Can you work these out from the drawing? Everything is in mm from the part's minimum corner. Coordinates: 2 decimals unless noted, no trailing zeros. Loops run counter-clockwise (first coordinate to the right, second up) from the corner with the lowest first, then second, coordinate; pieces in that order, holes last.
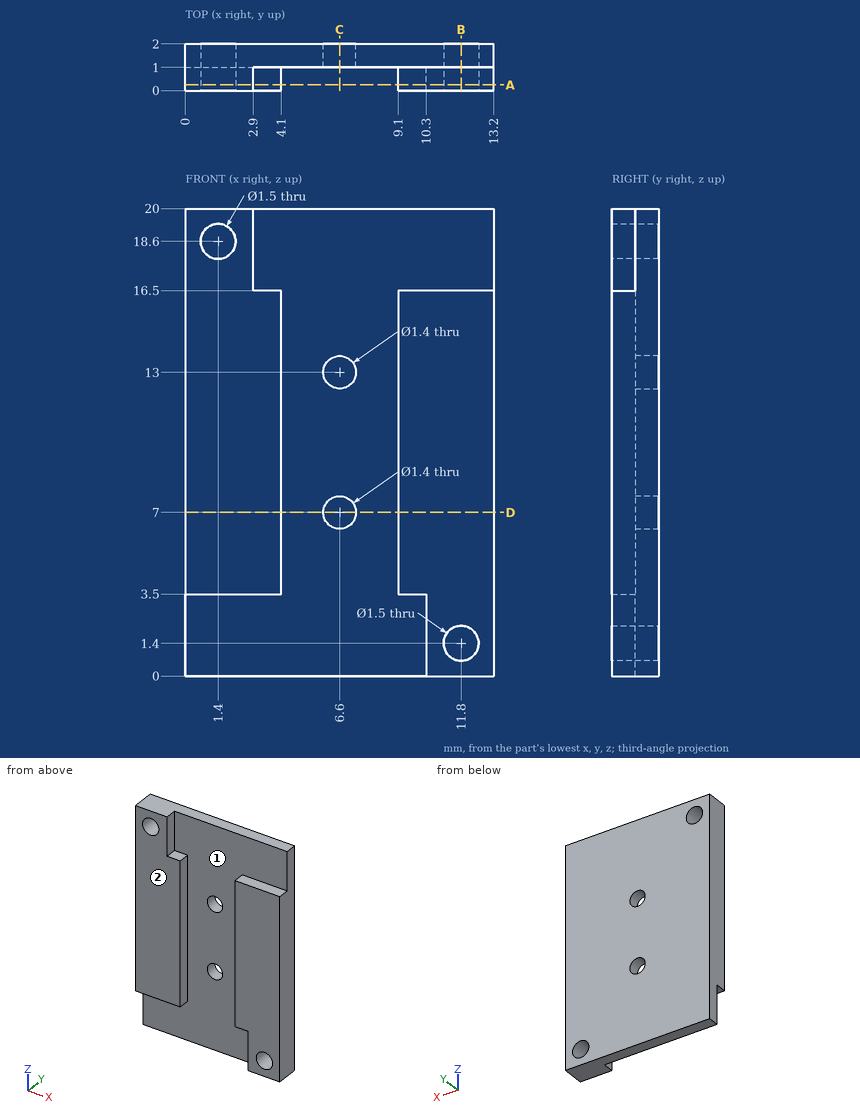
(1) For pin 1 (0.5 mm diameter, centred on y = 0.5, z = 2, fed in from -X); pin 2 (1.3 mm diameter, centred on x = 6.6, z = 7, fed in from +Y); pin 3 (0.5 mm diameter, centred on y = 0.5, z = 18.5, fed in from +X); pin 4 (0.5 mm diameter, centred on x = 11, y = 0.5, fed in from +Z), each with a flat end and sliding along its axis, tell me the tip position at first contact or that it passes through.
Answers:
pin 1: stops at x = 10.3
pin 2: passes through
pin 3: stops at x = 2.9
pin 4: stops at z = 16.5
(2) Imagine slicing it at A-A, the plane y = 0.25. Write out the boundary of the cut face in (x, z), and give its area (3 significant figures).
Answers:
outline: (0, 3.5) - (4.1, 3.5) - (4.1, 16.5) - (2.9, 16.5) - (2.9, 20) - (0, 20) - close; (9.1, 3.5) - (10.3, 3.5) - (10.3, 0) - (13.2, 0) - (13.2, 16.5) - (9.1, 16.5) - close; hole circle Ø1.5 at (1.4, 18.6); hole circle Ø1.5 at (11.8, 1.4)
area: 123 mm2
(3) I need wall thicknesses on probe 1 along X at (y, z) = (0.4, 12); probe 2 along X at (y, z) = (0.6, 1.4); probe 3 along Y at (x, z) = (5, 4.75). Which ranges of each line are inside material? Lowest first, please.
Answers:
probe 1: x = 0 to 4.1, 9.1 to 13.2
probe 2: x = 10.3 to 11.05, 12.55 to 13.2
probe 3: y = 1 to 2
(4) We'd pull the mould along X, two halves only. Please class the marked faces 1 and 2: +X half, -X half, draft (parallel to the pull), parting line (faces both ways), or undercut.
Answers:
face 1: undercut
face 2: draft
(5) Imagine slicing it at C-C, the plane x = 6.6. Write out the boundary of the cut face in (y, z).
Answers:
outline: (1, 0) - (2, 0) - (2, 6.3) - (1, 6.3) - close; (1, 7.7) - (2, 7.7) - (2, 12.3) - (1, 12.3) - close; (1, 13.7) - (2, 13.7) - (2, 20) - (1, 20) - close
(6) Imagine slicing it at B-B, the plane x = 11.8. Write out the boundary of the cut face in (y, z), and give its area (3 significant figures).
Answers:
outline: (0, 0) - (2, 0) - (2, 0.65) - (0, 0.65) - close; (0, 2.15) - (2, 2.15) - (2, 20) - (1, 20) - (1, 16.5) - (0, 16.5) - close
area: 33.5 mm2
(7) Imagine slicing it at D-D, the plane z = 7. Write out the boundary of the cut face in (x, y).
Answers:
outline: (0, 0) - (4.1, 0) - (4.1, 1) - (5.9, 1) - (5.9, 2) - (0, 2) - close; (7.3, 1) - (9.1, 1) - (9.1, 0) - (13.2, 0) - (13.2, 2) - (7.3, 2) - close
